Here's how the part is built. I have some questions about the finished solid (model axes, mm). Face numbers are marked on the shaded views. A direction names the side the tool comes from. Coordinates: 2 decimals unless noted, no trailing zeros. Write each loop counter-clockwise with the first axis right and the second up, starting at its lowest first coordinate (ties: lowest second). Pieces come first, ordered by that corner, then holes.
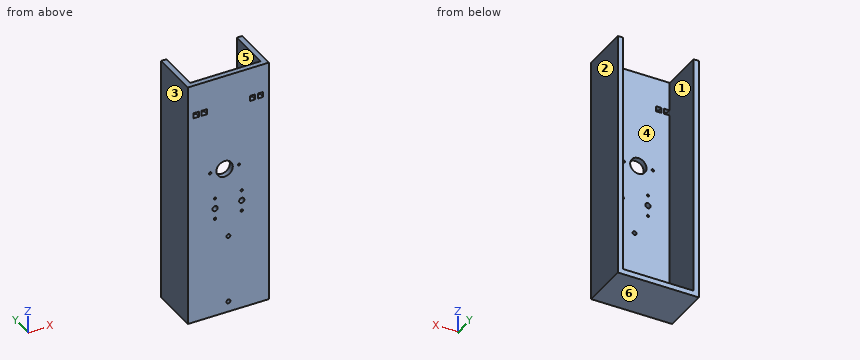
```python
from build123d import *

# Parameters (mm, degrees)
BOSS_EXTRUDE1_DEPTH            = 294.64
SKETCH2_W                      = 83.5
SKETCH2_H                      = 6.35
BOSS_EXTRUDE2_DEPTH            = 50.8
SKETCH3_R                      = 2.38125
CUT_EXTRUDE1_DEPTH             = 6.35
CUT_EXTRUDE2_REACH             = 304.832
SKETCH4_R                      = 9.7282
SKETCH4_R_2                    = 1.3890625
CUT_EXTRUDE3_REACH             = 304.832
SKETCH5_R                      = 3.175
SKETCH5_R_2                    = 1.3890625
CUT_EXTRUDE3_DIRECTION_2_DEPTH = 303.83160271
SKETCH6_W                      = 6.35
SKETCH6_H                      = 6.35
CUT_EXTRUDE4_DEPTH             = 6.35


with BuildPart() as part:
    # Sketch1 → Boss-Extrude1 (new body)
    with BuildSketch(Plane.XY):
        Polygon((0, 0), (41.75, 0), (41.75, 22.225), (41.75, 50.8), (48.1, 50.8), (48.1, -6.35), (0, -6.35), align=None)
    extrude(amount=BOSS_EXTRUDE1_DEPTH)

    # Mirror1: part across plane


with BuildPart() as part_1:
    add(part.part)
    add(part.part.mirror(Plane(origin=(0, -6.35, 294.64), x_dir=(0, 0, 1), z_dir=(-1, 0, 0))))

    # Sketch2 → Boss-Extrude2 (add)
    with BuildSketch(Plane(origin=(0, 0, 0), x_dir=(1, 0, 0), z_dir=(0, 1, 0))):
        with Locations((0, -3.175)):
            Rectangle(SKETCH2_W, SKETCH2_H)
    extrude(amount=BOSS_EXTRUDE2_DEPTH)

    # Sketch3 → Cut-Extrude1 (cut)
    with BuildSketch(Plane.XZ.offset(6.35)):
        with Locations((0, 12.7)):
            Circle(SKETCH3_R)
        with Locations((0, 93.98)):
            Circle(SKETCH3_R)
    extrude(amount=-CUT_EXTRUDE1_DEPTH, mode=Mode.SUBTRACT)

    # Sketch4 → Cut-Extrude2 (cut, up to next)
    with BuildSketch(Plane(origin=(0, 0, 0), x_dir=(1, 0, 0), z_dir=(0, 1, 0)), mode=Mode.PRIVATE) as cut_extrude2_sk1:
        with Locations(Location((-4.490010202, -179.209178053, 0), (0, 0, 270))):
            Circle(SKETCH4_R)
    cut_extrude2_tool1 = extrude(cut_extrude2_sk1.sketch, amount=-CUT_EXTRUDE2_REACH, mode=Mode.PRIVATE) & part_1.part
    # Sketch4 → Cut-Extrude2 (cut, up to next)
    with BuildSketch(Plane(origin=(0, 0, 0), x_dir=(1, 0, 0), z_dir=(0, 1, 0)), mode=Mode.PRIVATE) as cut_extrude2_sk2:
        with Locations(Location((-21.635010202, -179.209178053, 0), (0, 0, 270))):
            Circle(SKETCH4_R_2)
    cut_extrude2_tool2 = extrude(cut_extrude2_sk2.sketch, amount=-CUT_EXTRUDE2_REACH, mode=Mode.PRIVATE) & part_1.part
    # Sketch4 → Cut-Extrude2 (cut, up to next)
    with BuildSketch(Plane(origin=(0, 0, 0), x_dir=(1, 0, 0), z_dir=(0, 1, 0)), mode=Mode.PRIVATE) as cut_extrude2_sk3:
        with Locations(Location((12.654989798, -179.209178053, 0), (0, 0, 270))):
            Circle(SKETCH4_R_2)
    cut_extrude2_tool3 = extrude(cut_extrude2_sk3.sketch, amount=-CUT_EXTRUDE2_REACH, mode=Mode.PRIVATE) & part_1.part
    add(cut_extrude2_tool1.solids().sort_by_distance((-4.49001, 0, 179.209178))[0], mode=Mode.SUBTRACT)
    add(cut_extrude2_tool2.solids().sort_by_distance((-21.63501, 0, 179.209178))[0], mode=Mode.SUBTRACT)
    add(cut_extrude2_tool3.solids().sort_by_distance((12.65499, 0, 179.209178))[0], mode=Mode.SUBTRACT)

    # Sketch5 → Cut-Extrude3 (cut, up to next)
    with BuildSketch(Plane(origin=(0, 0, 0), x_dir=(1, 0, 0), z_dir=(0, 1, 0)), mode=Mode.PRIVATE) as cut_extrude3_sk1:
        with Locations((15.8749986, -133.35)):
            Circle(SKETCH5_R)
    cut_extrude3_tool1 = extrude(cut_extrude3_sk1.sketch, amount=-CUT_EXTRUDE3_REACH, mode=Mode.PRIVATE) & part_1.part
    # Sketch5 → Cut-Extrude3 (cut, up to next)
    with BuildSketch(Plane(origin=(0, 0, 0), x_dir=(1, 0, 0), z_dir=(0, 1, 0)), mode=Mode.PRIVATE) as cut_extrude3_sk2:
        with Locations((-15.8749986, -133.35)):
            Circle(SKETCH5_R)
    cut_extrude3_tool2 = extrude(cut_extrude3_sk2.sketch, amount=-CUT_EXTRUDE3_REACH, mode=Mode.PRIVATE) & part_1.part
    # Sketch5 → Cut-Extrude3 (cut, up to next)
    with BuildSketch(Plane(origin=(0, 0, 0), x_dir=(1, 0, 0), z_dir=(0, 1, 0)), mode=Mode.PRIVATE) as cut_extrude3_sk3:
        with Locations((15.8749986, -146.05)):
            Circle(SKETCH5_R_2)
    cut_extrude3_tool3 = extrude(cut_extrude3_sk3.sketch, amount=-CUT_EXTRUDE3_REACH, mode=Mode.PRIVATE) & part_1.part
    # Sketch5 → Cut-Extrude3 (cut, up to next)
    with BuildSketch(Plane(origin=(0, 0, 0), x_dir=(1, 0, 0), z_dir=(0, 1, 0)), mode=Mode.PRIVATE) as cut_extrude3_sk4:
        with Locations((15.8749986, -120.65)):
            Circle(SKETCH5_R_2)
    cut_extrude3_tool4 = extrude(cut_extrude3_sk4.sketch, amount=-CUT_EXTRUDE3_REACH, mode=Mode.PRIVATE) & part_1.part
    # Sketch5 → Cut-Extrude3 (cut, up to next)
    with BuildSketch(Plane(origin=(0, 0, 0), x_dir=(1, 0, 0), z_dir=(0, 1, 0)), mode=Mode.PRIVATE) as cut_extrude3_sk5:
        with Locations((-15.8749986, -146.05)):
            Circle(SKETCH5_R_2)
    cut_extrude3_tool5 = extrude(cut_extrude3_sk5.sketch, amount=-CUT_EXTRUDE3_REACH, mode=Mode.PRIVATE) & part_1.part
    # Sketch5 → Cut-Extrude3 (cut, up to next)
    with BuildSketch(Plane(origin=(0, 0, 0), x_dir=(1, 0, 0), z_dir=(0, 1, 0)), mode=Mode.PRIVATE) as cut_extrude3_sk6:
        with Locations((-15.8749986, -120.65)):
            Circle(SKETCH5_R_2)
    cut_extrude3_tool6 = extrude(cut_extrude3_sk6.sketch, amount=-CUT_EXTRUDE3_REACH, mode=Mode.PRIVATE) & part_1.part
    add(cut_extrude3_tool1.solids().sort_by_distance((15.874999, 0, 133.35))[0], mode=Mode.SUBTRACT)
    add(cut_extrude3_tool2.solids().sort_by_distance((-15.874999, 0, 133.35))[0], mode=Mode.SUBTRACT)
    add(cut_extrude3_tool3.solids().sort_by_distance((15.874999, 0, 146.05))[0], mode=Mode.SUBTRACT)
    add(cut_extrude3_tool4.solids().sort_by_distance((15.874999, 0, 120.65))[0], mode=Mode.SUBTRACT)
    add(cut_extrude3_tool5.solids().sort_by_distance((-15.874999, 0, 146.05))[0], mode=Mode.SUBTRACT)
    add(cut_extrude3_tool6.solids().sort_by_distance((-15.874999, 0, 120.65))[0], mode=Mode.SUBTRACT)

    # Sketch5 → Cut-Extrude3 direction 2 (cut)
    with BuildSketch(Plane(origin=(0, 0, 0), x_dir=(1, 0, 0), z_dir=(0, 1, 0))):
        with Locations((15.8749986, -133.35)):
            Circle(SKETCH5_R)
        with Locations((-15.8749986, -133.35)):
            Circle(SKETCH5_R)
        with Locations((15.8749986, -146.05)):
            Circle(SKETCH5_R_2)
        with Locations((15.8749986, -120.65)):
            Circle(SKETCH5_R_2)
        with Locations((-15.8749986, -146.05)):
            Circle(SKETCH5_R_2)
        with Locations((-15.8749986, -120.65)):
            Circle(SKETCH5_R_2)
    extrude(amount=CUT_EXTRUDE3_DIRECTION_2_DEPTH, mode=Mode.SUBTRACT)

    # Sketch6 → Cut-Extrude4 (cut)
    with BuildSketch(Plane(origin=(0, 0, 0), x_dir=(1, 0, 0), z_dir=(0, 1, 0))):
        with Locations((28.575, -257.175)):
            Rectangle(SKETCH6_W, SKETCH6_H)
        with Locations((-28.575, -257.175)):
            Rectangle(SKETCH6_W, SKETCH6_H)
        with Locations((38.1, -257.175)):
            Rectangle(SKETCH6_W, SKETCH6_H)
        with Locations((-38.1, -257.175)):
            Rectangle(SKETCH6_W, SKETCH6_H)
    extrude(amount=-CUT_EXTRUDE4_DEPTH, mode=Mode.SUBTRACT)


solid = part_1.part
```
1) On a 3-axis mill with a long thin cutter (end or side, diameter ignored), from which of +Z, -Z, +X, -X, +Y, -Y can I reach the whole of each face in a straight line? I mean the marked faces 5 and 6. Say none if no direction works.
Values follow:
face 5: +Z, +Y
face 6: -Z, +X, -X, +Y, -Y
2) I need wall thicknesses on probe 1 along X at (y, z) = (-4, 120.65); probe 2 along X at (y, z) = (27.5, 94); probe 3 along X at (y, z) = (-2, 120). Which ranges of each line are inside material? Lowest first, please.
Values follow:
probe 1: x = -48.1 to -17.26, -14.49 to 14.49, 17.26 to 48.1
probe 2: x = -48.1 to -41.75, 41.75 to 48.1
probe 3: x = -48.1 to -17.1, -14.65 to 14.65, 17.1 to 48.1
3) Will these pins go through, and if not, where does the flat tip stop? pin 1 (5.5 mm diameter, centred on x = 0, z = 93.98, fed in from +Y); pin 2 (1.5 mm diameter, centred on x = -18.5, y = 23.5, fed in from +Z).
Values follow:
pin 1: stops at y = 0
pin 2: stops at z = 6.35
4) Imagine slicing it at A-A on z = 133.35. Please give me the cut outline in (x, y), then the cut area to 3 significant figures.
Values follow:
outline: (-48.1, -6.35) - (-19.05, -6.35) - (-19.05, 0) - (-41.75, 0) - (-41.75, 50.8) - (-48.1, 50.8) - close; (-12.7, -6.35) - (12.7, -6.35) - (12.7, 0) - (-12.7, 0) - close; (19.05, -6.35) - (48.1, -6.35) - (48.1, 50.8) - (41.75, 50.8) - (41.75, 0) - (19.05, 0) - close
area: 1,180 mm2
5) We'd pull the mould along X, two halves only. Please class the marked faces 1, 2, 3 and 4: pulls with the +X half, pulls with the -X half, needs draft (parallel to the pull), parting line crosses it, or undercut.
Values follow:
face 1: undercut
face 2: pulls with the +X half
face 3: pulls with the -X half
face 4: undercut
6) Imagine slicing it at B-B on y = 44. Please give me the cut outline in (x, z).
Values follow:
outline: (-48.1, 0) - (48.1, 0) - (48.1, 294.64) - (41.75, 294.64) - (41.75, 6.35) - (-41.75, 6.35) - (-41.75, 294.64) - (-48.1, 294.64) - close
